from build123d import *

# Parameters (mm, degrees)
SKETCH011_W  = 95.2
SKETCH011_H  = 12.9
PAD009_DEPTH = 30
FILLET002_R  = 3
PAD008_DEPTH = 161.6


with BuildPart() as tubecutout001:
    # Sketch011 → Pad009 (new body)
    with BuildSketch(Plane(origin=(-10.7, 54, 33), x_dir=(1, 0, 0), z_dir=(0, -1, 0))):
        Rectangle(SKETCH011_W, SKETCH011_H)
    extrude(amount=PAD009_DEPTH)

    # Fillet002
    fillet002_edges = [tubecutout001.edges().sort_by_distance(p)[0] for p in [
        (-58.3, 39, 39.45),
        (-58.3, 39, 26.55),
        (36.9, 39, 39.45),
        (36.9, 39, 26.55),
    ]]
    fillet(fillet002_edges, radius=FILLET002_R)


with BuildPart() as boxcover:
    # Sketch010 → Pad008 (new body)
    with BuildSketch(Plane(origin=(-81, 0, 25.5), x_dir=(0, 1, 0), z_dir=(1, 0, 0))):
        Polygon((-43.55, -25.6), (-43.55, 28), (43.55, 28), (43.55, -25.6), (41.15, -25.6), (41.15, 25.6), (-41.15, 25.6), (-41.15, -25.6), align=None)
    extrude(amount=PAD008_DEPTH)

    # Cut001: cut TubeCutout001
    add(tubecutout001.part, mode=Mode.SUBTRACT)


solid = boxcover.part
CAD build for the part. Positions are in the model's coordinates, mm. A direction names the side the tool comes from. Round coordinates to 2 decimals unless told otherwise and drop trailing zeros. Order: outer loops, then holes, each group sorted by start corner. A loop starts at its lowest first (then second) coordinate and runs counter-clockwise, first axis right, second up. Notation, with made-up numbers: (-18, -18.75) -> (32, -18.75) arc R17 ccw to (32, -10.75) -> close; hole circle Ø7 at (-26.5, 0.5). An arc over 180 degrees is marked (long way). Write item = value, one per line. Start each with the question number.
(1) Pull direction Z, two halves, no side cores. Call faces 1 (the flat face through (-1, -43.55, 26)), 2 (the cylindrical face through (-57.44, 42.33, 27.45)), 3 (the flat face through (-1, 1, 51.1)): released by +Z, released by -Z, zero draft, split by the parting line, or undercut.
(2) Cut at B-B, the plane z = 34.5. List the corners of the cut face in (x, y), then the cut area to 3 significant figures.
(3) Probe line 1 (Y direction, x = 35, z = 3.5); line 2 (Y direction, x = 23, z = 29); line 3 (Z direction, x = -1, y = 4). List the from-to ranges inside material, lowest first. Write a range as [from, to].
(4) Pin check, flat tip, straight feed: P1, Ø10, axis at x = 25.5, y = -22.5, coming from the -Z side. Stop position of the tip, or through.
(5) Cut at D-D, the plane x = 39. List the corners of the cut face in (y, z).
(6) Cut at A-A, the plane x = -2. List the corners of the cut face in (y, z), then the cut area to 3 significant figures.
(7) Which spindle directions (+Z, -Z, +X, -X, +Y, -Y) get a long thin tool onto all of the face, cutting with end or side? Do faces 4 (the flat face through (-1, -1, 53.5)), 5 (the cylindrical face through (36.04, 42.33, 38.55)), 6 (the flat face through (-1, 41.15, 25)). Say none if no direction does.
(8) Cut at C-C, the plane z = 17. List the corners of the cut face in (x, y).
Model answer:
q1.face_1 = zero draft
q1.face_2 = undercut
q1.face_3 = released by -Z
q2.outline = (-81, -43.55) -> (80.6, -43.55) -> (80.6, -41.15) -> (-81, -41.15) -> close; (-81, 41.15) -> (-58.3, 41.15) -> (-58.3, 43.55) -> (-81, 43.55) -> close; (36.9, 41.15) -> (80.6, 41.15) -> (80.6, 43.55) -> (36.9, 43.55) -> close
q2.area = 547 mm2
q3.line_1 = [-43.55, -41.15], [41.15, 43.55]
q3.line_2 = [-43.55, -41.15]
q3.line_3 = [51.1, 53.5]
q4.P1 = 51.1
q5.outline = (-43.55, -0.1) -> (-41.15, -0.1) -> (-41.15, 51.1) -> (41.15, 51.1) -> (41.15, -0.1) -> (43.55, -0.1) -> (43.55, 53.5) -> (-43.55, 53.5) -> close
q6.outline = (-43.55, -0.1) -> (-41.15, -0.1) -> (-41.15, 51.1) -> (41.15, 51.1) -> (41.15, 39.45) -> (43.55, 39.45) -> (43.55, 53.5) -> (-43.55, 53.5) -> close; (41.15, -0.1) -> (43.55, -0.1) -> (43.55, 26.55) -> (41.15, 26.55) -> close
q6.area = 424 mm2
q7.face_4 = +Z, +X, -X, +Y, -Y
q7.face_5 = +Y
q7.face_6 = -Z, +X, -X
q8.outline = (-81, -43.55) -> (80.6, -43.55) -> (80.6, -41.15) -> (-81, -41.15) -> close; (-81, 41.15) -> (80.6, 41.15) -> (80.6, 43.55) -> (-81, 43.55) -> close
